```python
from build123d import *

# Parameters (mm, degrees)
SKETCH2_R           = 2.778125
BOSS_EXTRUDE1_DEPTH = 6.35
CUT_EXTRUDE1_DEPTH  = 280.596929737
FILLET1_R           = 2.54


with BuildPart() as part:
    # Sketch2 → Boss-Extrude1 (new body)
    with BuildSketch(Plane.XY):
        with BuildLine():
            Line((25.4, 2.542062626), (76.2, 2.542062626))
            Line((76.2, 2.542062626), (76.2, 5.717062626))
            Line((76.2, 5.717062626), (152.4, 5.717062626))
            Line((152.4, 5.717062626), (152.4, 2.542062626))
            Line((152.4, 2.542062626), (177.8, 2.542062626))
            Line((177.8, 2.542062626), (177.8, -3.807937374))
            Line((177.8, -3.807937374), (196.85, -3.807937374))
            Line((196.85, -3.807937374), (196.85, 78.742062626))
            Line((196.85, 78.742062626), (203.2, 78.742062626))
            Line((203.2, 78.742062626), (203.2, 104.142062626))
            Line((203.2, 104.142062626), (196.85, 104.142062626))
            Line((196.85, 104.142062626), (196.85, 129.542062626))
            Line((196.85, 129.542062626), (139.204596213, 186.076487834))
            ThreePointArc((139.204596213, 186.076487834), (122.208232851, 191.779061014), (107.214428724, 181.951469947))
            Line((107.214428724, 181.951469947), (0, 2.542062626))
            Line((0, 2.542062626), (0, -3.807937374))
            Line((0, -3.807937374), (25.4, -3.807937374))
            Line((25.4, -3.807937374), (25.4, 2.542062626))
        make_face()
        with Locations((124.833126, 171.422598626)):
            Circle(SKETCH2_R, mode=Mode.SUBTRACT)
    extrude(amount=BOSS_EXTRUDE1_DEPTH)

    # Sketch4 → Cut-Extrude1 (cut, through all)
    with BuildSketch(Plane.XY.offset(6.35)):
        with BuildLine():
            ThreePointArc((113.815309866, 160.551532388), (112.421969705, 162.174055338), (111.26558656, 163.973153877))
            Line((111.26558656, 163.973153877), (95.241664491, 137.159203595))
            Line((95.241664491, 137.159203595), (108.075962418, 116.386657845))
            Line((108.075962418, 116.386657845), (113.815309866, 160.551532388))
        make_face()
        with BuildLine():
            Line((160.218857543, 136.71884322), (135.883782706, 160.584917146))
            ThreePointArc((135.883782706, 160.584917146), (134.376571421, 159.23674605), (132.706463437, 158.096574796))
            Line((132.706463437, 158.096574796), (126.50513789, 110.376730818))
            Line((126.50513789, 110.376730818), (160.218857543, 136.71884322))
        make_face()
        Polygon((101.478261059, 90.822056657), (84.231843224, 118.735699112), (37.832728657, 41.092813319), align=None)
        Polygon((184.15, 113.248916833), (173.938776136, 123.263343551), (128.409628791, 87.689282626), (184.15, 31.894074467), align=None)
        Polygon((101.62722196, 66.762930434), (39.752190498, 18.417062626), (95.344542887, 18.417062626), align=None)
        Polygon((170.686233709, 18.417062626), (121.01587543, 68.136286224), (114.554724978, 18.417062626), align=None)
    extrude(amount=-CUT_EXTRUDE1_DEPTH, mode=Mode.SUBTRACT)

    # Fillet1
    # the kernel refuses this fillet: 2.54 mm, written as the material it adds along each edge
    with BuildSketch(Plane(origin=(101.478261059, 90.822056657, 6.35), x_dir=(-0.787987305363456, -0.6156914865304209, 0), z_dir=(0, 0, -1))) as fillet1_piece_1:
        with BuildLine():
            CenterArc((FILLET1_R * 0.89579463255, FILLET1_R), FILLET1_R, 186.292375304, 83.707624696)
            Line((-FILLET1_R * 0.0981809171118, FILLET1_R * 0.890397962274), (0, 0))
            Line((0, 0), (FILLET1_R * 0.89579463255, 0))
        make_face()
    extrude(amount=6.35)
    with BuildSketch(Plane(origin=(37.832728657, 41.092813319, 6.35), x_dir=(0.7879873053634544, 0.615691486530423, 0), z_dir=(0, 0, -1))) as fillet1_piece_2:
        with BuildLine():
            CenterArc((FILLET1_R * 5.36015588483, -FILLET1_R), FILLET1_R, 90, 158.864572417)
            Line((FILLET1_R * 4.9995822743, -FILLET1_R * 1.9327307604), (0, 0))
            Line((0, 0), (FILLET1_R * 5.36015588483, 0))
        make_face()
    extrude(amount=6.35)
    with BuildSketch(Plane(origin=(84.231843224, 118.735699112, 6.35), x_dir=(0.5256172693760891, -0.8507211565099483, 0), z_dir=(0, 0, -1))) as fillet1_piece_3:
        with BuildLine():
            CenterArc((FILLET1_R * 1.64561036796, FILLET1_R), FILLET1_R, 152.572197113, 117.427802887)
            Line((FILLET1_R * 0.758018400173, FILLET1_R * 1.46063054471), (0, 0))
            Line((0, 0), (FILLET1_R * 1.64561036796, 0))
        make_face()
    extrude(amount=6.35)
    with BuildSketch(Plane(origin=(111.26558656, 163.973153877, 6.35), x_dir=(-0.5129778962436395, -0.8584018161475719, 0), z_dir=(0, 0, -1))) as fillet1_piece_4:
        with BuildLine():
            CenterArc((3.871144204, -2.54), FILLET1_R, 90, 107.056570321)
            ThreePointArc((1.442864529, -3.285022026), (0.816940233, -1.600561505), (0, 0))
            Line((0, 0), (3.871144204, 0))
        make_face()
    extrude(amount=6.35)
    with BuildSketch(Plane(origin=(113.815309866, 160.551532388, 6.35), x_dir=(-0.12886916491369038, -0.9916616047495476, 0), z_dir=(0, 0, -1))) as fillet1_piece_5:
        with BuildLine():
            CenterArc((1.182123264, 2.54), FILLET1_R, 222.036471985, 47.963528015)
            ThreePointArc((-0.704382325, 0.839207048), (-0.344763298, 0.425838049), (0, 0))
            Line((0, 0), (1.182123264, 0))
        make_face()
    extrude(amount=6.35)
    with BuildSketch(Plane(origin=(108.075962418, 116.386657845, 6.35), x_dir=(-0.5256172693760838, 0.8507211565099515, 0), z_dir=(0, 0, -1))) as fillet1_piece_6:
        with BuildLine():
            CenterArc((FILLET1_R * 2.81500526937, FILLET1_R), FILLET1_R, 129.114057402, 140.885942598)
            Line((FILLET1_R * 2.18413907953, FILLET1_R * 1.77589164869), (0, 0))
            Line((0, 0), (FILLET1_R * 2.81500526937, 0))
        make_face()
    extrude(amount=6.35)
    with BuildSketch(Plane(origin=(95.241664491, 137.159203595, 6.35), x_dir=(0.5129778962436408, 0.8584018161475709, 0), z_dir=(0, 0, -1))) as fillet1_piece_7:
        with BuildLine():
            CenterArc((FILLET1_R * 0.607677260346, FILLET1_R), FILLET1_R, 207.427802887, 62.572197113)
            Line((-FILLET1_R * 0.279914707441, FILLET1_R * 0.539369455291), (0, 0))
            Line((0, 0), (FILLET1_R * 0.607677260346, 0))
        make_face()
    extrude(amount=6.35)
    with BuildSketch(Plane(origin=(39.752190498, 18.417062626, 6.35), x_dir=(0.787987305363458, 0.6156914865304186, 0), z_dir=(0, 0, -1))) as fillet1_piece_8:
        with BuildLine():
            CenterArc((FILLET1_R * 2.9040312307, FILLET1_R), FILLET1_R, 128.002182129, 141.997817871)
            Line((FILLET1_R * 2.28833974417, FILLET1_R * 1.78798730536), (0, 0))
            Line((0, 0), (FILLET1_R * 2.9040312307, 0))
        make_face()
    extrude(amount=6.35)
    with BuildSketch(Plane(origin=(101.62722196, 66.762930434, 6.35), x_dir=(-0.7879873053634603, -0.6156914865304155, 0), z_dir=(0, 0, -1))) as fillet1_piece_9:
        with BuildLine():
            CenterArc((FILLET1_R * 2.438641865, -FILLET1_R), FILLET1_R, 90, 135.406432707)
            Line((FILLET1_R * 1.73656875695, -FILLET1_R * 1.71210487357), (0, 0))
            Line((0, 0), (FILLET1_R * 2.438641865, 0))
        make_face()
    extrude(amount=6.35)
    with BuildSketch(Plane(origin=(95.344542887, 18.417062626, 6.35), x_dir=(-1, 0, 0), z_dir=(0, 0, -1))) as fillet1_piece_10:
        with BuildLine():
            CenterArc((FILLET1_R * 0.878455746309, FILLET1_R), FILLET1_R, 187.404250578, 82.595749422)
            Line((-FILLET1_R * 0.11320585844, FILLET1_R * 0.871130835086), (0, 0))
            Line((0, 0), (FILLET1_R * 0.878455746309, 0))
        make_face()
    extrude(amount=6.35)
    with BuildSketch(Plane(origin=(121.01587543, 68.136286224, 6.35), x_dir=(0.7067590436590283, -0.7074543477894356, 0), z_dir=(0, 0, -1))) as fillet1_piece_11:
        with BuildLine():
            CenterArc((FILLET1_R * 2.03333963012, FILLET1_R), FILLET1_R, 142.376080862, 127.623919138)
            Line((FILLET1_R * 1.2413047717, FILLET1_R * 1.61047586606), (0, 0))
            Line((0, 0), (FILLET1_R * 2.03333963012, 0))
        make_face()
    extrude(amount=6.35)
    with BuildSketch(Plane(origin=(170.686233709, 18.417062626, 6.35), x_dir=(-1, 0, 0), z_dir=(0, 0, -1))) as fillet1_piece_12:
        with BuildLine():
            CenterArc((FILLET1_R * 2.41253594524, FILLET1_R), FILLET1_R, 135.028169716, 134.971830284)
            Line((FILLET1_R * 1.70508159745, FILLET1_R * 1.70675904366), (0, 0))
            Line((0, 0), (FILLET1_R * 2.41253594524, 0))
        make_face()
    extrude(amount=6.35)
    with BuildSketch(Plane(origin=(114.554724978, 18.417062626, 6.35), x_dir=(1, 0, 0), z_dir=(0, 0, -1))) as fillet1_piece_13:
        with BuildLine():
            CenterArc((FILLET1_R * 1.13836127113, -FILLET1_R), FILLET1_R, 90, 97.404250578)
            Line((FILLET1_R * 0.14669966638, -FILLET1_R * 1.12886916491), (0, 0))
            Line((0, 0), (FILLET1_R * 1.13836127113, 0))
        make_face()
    extrude(amount=6.35)
    with BuildSketch(Plane(origin=(132.706463437, 158.096574796, 6.35), x_dir=(-0.12886916491355233, -0.9916616047495656, 0), z_dir=(0, 0, -1))) as fillet1_piece_14:
        with BuildLine():
            CenterArc((1.182123264, -2.54), FILLET1_R, 90, 47.963528015)
            ThreePointArc((-0.704382325, -0.839207048), (-0.344763298, -0.425838049), (0, 0))
            Line((0, 0), (1.182123264, 0))
        make_face()
    extrude(amount=6.35)
    with BuildSketch(Plane(origin=(135.883782706, 160.584917146, 6.35), x_dir=(0.7139531891838808, -0.7001934330270213, 0), z_dir=(0, 0, -1))) as fillet1_piece_15:
        with BuildLine():
            CenterArc((2.360070775, 2.54), FILLET1_R, 188.103931403, 81.896068597)
            ThreePointArc((-0.154564753, 2.181938326), (-0.038689543, 1.093703013), (0, 0))
            Line((0, 0), (2.360070775, 0))
        make_face()
    extrude(amount=6.35)
    with BuildSketch(Plane(origin=(160.218857543, 136.71884322, 6.35), x_dir=(-0.7879873053634604, -0.6156914865304155, 0), z_dir=(0, 0, -1))) as fillet1_piece_16:
        with BuildLine():
            CenterArc((FILLET1_R * 1.14139198058, FILLET1_R), FILLET1_R, 172.444707349, 97.555292651)
            Line((FILLET1_R * 0.150073543693, FILLET1_R * 1.13148291406), (0, 0))
            Line((0, 0), (FILLET1_R * 1.14139198058, 0))
        make_face()
    extrude(amount=6.35)
    with BuildSketch(Plane(origin=(126.50513789, 110.376730818, 6.35), x_dir=(0.1288691649135192, 0.9916616047495699, 0), z_dir=(0, 0, -1))) as fillet1_piece_17:
        with BuildLine():
            CenterArc((FILLET1_R * 2.438641865, FILLET1_R), FILLET1_R, 134.593567293, 135.406432707)
            Line((FILLET1_R * 1.73656875695, FILLET1_R * 1.71210487357), (0, 0))
            Line((0, 0), (FILLET1_R * 2.438641865, 0))
        make_face()
    extrude(amount=6.35)
    with BuildSketch(Plane(origin=(184.15, 113.248916833, 6.35), x_dir=(0, -1, 0), z_dir=(0, 0, -1))) as fillet1_piece_18:
        with BuildLine():
            CenterArc((FILLET1_R * 0.41992468346, FILLET1_R), FILLET1_R, 224.44252522, 45.55747478)
            Line((-FILLET1_R * 0.294028505724, FILLET1_R * 0.299806566973), (0, 0))
            Line((0, 0), (FILLET1_R * 0.41992468346, 0))
        make_face()
    extrude(amount=6.35)
    with BuildSketch(Plane(origin=(184.15, 31.894074467, 6.35), x_dir=(-0.7067590436590262, 0.7074543477894377, 0), z_dir=(0, 0, -1))) as fillet1_piece_19:
        with BuildLine():
            CenterArc((FILLET1_R * 2.41589317195, FILLET1_R), FILLET1_R, 134.971830284, 135.028169716)
            Line((FILLET1_R * 1.70913412829, FILLET1_R * 1.70745434779), (0, 0))
            Line((0, 0), (FILLET1_R * 2.41589317195, 0))
        make_face()
    extrude(amount=6.35)
    with BuildSketch(Plane(origin=(128.409628791, 87.689282626, 6.35), x_dir=(0.7879873053634587, 0.6156914865304174, 0), z_dir=(0, 0, -1))) as fillet1_piece_20:
        with BuildLine():
            CenterArc((FILLET1_R * 1.12969130859, FILLET1_R), FILLET1_R, 173.030351844, 96.969648156)
            Line((FILLET1_R * 0.137080737194, FILLET1_R * 1.12134353531), (0, 0))
            Line((0, 0), (FILLET1_R * 1.12969130859, 0))
        make_face()
    extrude(amount=6.35)
    with BuildSketch(Plane(origin=(173.938776136, 123.263343551, 6.35), x_dir=(-0.7879873053634626, -0.6156914865304124, 0), z_dir=(0, 0, -1))) as fillet1_piece_21:
        with BuildLine():
            CenterArc((FILLET1_R * 0.876123204837, -FILLET1_R), FILLET1_R, 90, 82.444707349)
            Line((-FILLET1_R * 0.115195232049, -FILLET1_R * 0.868517085939), (0, 0))
            Line((0, 0), (FILLET1_R * 0.876123204837, 0))
        make_face()
    extrude(amount=6.35)


solid = part.part
```
Geometry check sheet. Reference: the model listing, model coordinates, mm. A direction names the side the tool comes from. Give positions to 0.01 mm unless a question says otherwise; leave off trailing zeros. Write each loop counter-clockwise with the first axis right and the second up, starting at its lowest first coordinate (ties: lowest second). Pieces come first, ordered by that corner, then holes. Notation, with made-up numbers: (48, -6) -> (77, -6) arc R25 ccw to (77, 32) -> close; hole circle Ø5 at (51, 70.25). An arc over 180 degrees is marked (long way). One line per question, with ' | ' between items.
Item 1: Sectioned sample at A-A, the plane x = 79.5. Record the boundary of the cut face in (y, z).
Determined:
outline: (5.72, 0) -> (18.42, 0) -> (18.42, 6.35) -> (5.72, 6.35) -> close; (49.47, 0) -> (73.65, 0) -> (73.65, 6.35) -> (49.47, 6.35) -> close; (110.82, 0) -> (135.57, 0) -> (135.57, 6.35) -> (110.82, 6.35) -> close
Item 2: Sectioned sample at D-D, the plane x = 18.5. Record the boundary of the cut face in (y, z).
Determined:
outline: (-3.81, 0) -> (33.5, 0) -> (33.5, 6.35) -> (-3.81, 6.35) -> close
Item 3: Sectioned sample at B-B, the plane y = 142. Record the boundary of the cut face in (x, z), plus the area to 3 significant figures.
Determined:
outline: (83.34, 0) -> (98.13, 0) -> (98.13, 6.35) -> (83.34, 6.35) -> close; (111.4, 0) -> (130.61, 0) -> (130.61, 6.35) -> (111.4, 6.35) -> close; (154.83, 0) -> (184.15, 0) -> (184.15, 6.35) -> (154.83, 6.35) -> close | area: 402 mm^2
Item 4: Scan lines: line 1 along Y through (x, z) = (61, 0.5); line 2 along X through (y, z) = (91.5, 3.25); line 3 along X through (y, z) = (151.5, 3). Record each from-to range of solid material in increasing order.
Determined:
line 1: 2.54 to 18.42, 35.02 to 59.19, 79.86 to 104.62 | line 2: 53.16 to 67.96, 100.66 to 133.29, 184.15 to 203.2 | line 3: 89.02 to 103.81, 112.64 to 131.85, 145.15 to 174.46
Item 5: Draft check along Y on faces 5 (the flat face through (177.8, -1, 3)), 6 (the flat face through (73.77, 69.17, 3.22)), 7 (the flat face through (54.358, 93.503, 3.131)). Enter one of: released by +Y, released by -Y, zero draft, split by the parting line, or undercut.
Determined:
face 5: zero draft | face 6: undercut | face 7: released by +Y
Item 6: Sectioned sample at C-C, the plane z = 1. State how many separate pieces and enclosed holes the cut face has, plus the area to 3 significant figures.
Determined:
separate pieces: 1 | enclosed holes: 7 | area: 16,900 mm^2
Item 7: Depth check by flat-ended pin: pin 1 (1 mm diameter, centred on y = 3.5, z = 4, fed in from -X); pin 2 (1.9 mm diameter, centred on x = 200.5, z = 1.5, fed in from -Y); pin 3 (3 mm diameter, centred on y = 0.5, z = 3.5, fed in from +X); pin 4 (5 mm diameter, centred on x = 124.83, y = 171.42, fed in from -Z). Enter the tip coordinate at first touch or a pass-through.
Determined:
pin 1: x = 0.27 | pin 2: y = 78.74 | pin 3: x = 196.85 | pin 4: through
Item 8: Access from +Z, -Z, +X, -X, +Y, -Y to the whole of each face (thin tool, end or side, straight path). Record for faces 1 (the flat face through (179.51, 117.8, 3.22)), 2 (the flat face through (200, 78.742, 3)), 3 (the cylindrical face through (122.47, 191.81, 3.13)), 4 (the flat face through (114, 5.717, 3)).
Determined:
face 1: +Z, -Z | face 2: +Z, -Z, +X, -Y | face 3: +Z, -Z, +Y | face 4: +Z, -Z, -Y
